The listing builds one solid part. Answer for the finished solid, in the listing's coordinates (mm). A direction names the side the tool comes from. Coordinates: 2 decimals unless noted, no trailing zeros. Order: outer loops, then holes, each group sorted by start corner. A loop starts at its lowest first (then second) coordinate and runs counter-clockwise, first axis right, second up. Notation, with made-up numbers: (48, -38) -> (54, -38) arc R26 ccw to (54, -24) -> close; hole circle Ø10 at (51, -20.75). An arc over 180 degrees is marked (long way). Write item = value, one per line.
from build123d import *

# Parameters (mm, degrees)
F0_W     = 23.8
F0_H     = 14
F0_W_2   = 10.5
F0_H_2   = 12
F1_DEPTH = 5.5
F2_DEPTH = 1.5
F4_DEPTH = 1
F5_R     = 6.5


with BuildPart() as f1:
    # F0 (on Top) → F1 (new body)
    with BuildSketch(Plane.XY):
        with Locations((-0.285932, 2.603267)):
            Rectangle(F0_W, F0_H)
        with Locations((-5.935932, 2.603267)):
            Rectangle(F0_W_2, F0_H_2, mode=Mode.SUBTRACT)
        with BuildLine():
            ThreePointArc((4.464068, 7.655247), (5.464068, 7.753267), (6.464068, 7.655247))
            ThreePointArc((6.464068, 7.655247), (9.443546, 5.87225), (10.614068, 2.603267))
            ThreePointArc((10.614068, 2.603267), (9.443546, -0.665716), (6.464068, -2.448713))
            ThreePointArc((6.464068, -2.448713), (5.464068, -2.546733), (4.464068, -2.448713))
            ThreePointArc((4.464068, -2.448713), (0.314068, 2.603267), (4.464068, 7.655247))
        make_face(mode=Mode.SUBTRACT)
    extrude(amount=F1_DEPTH)

    # F0 (on Top) → F2 (join)
    with BuildSketch(Plane.XY):
        with BuildLine():
            Line((4.464068, 4.655247), (6.464068, 4.655247))
            Line((6.464068, 4.655247), (6.464068, 7.655247))
            ThreePointArc((6.464068, 7.655247), (5.464068, 7.753267), (4.464068, 7.655247))
            Line((4.464068, 7.655247), (4.464068, 4.655247))
        make_face()
        with BuildLine():
            ThreePointArc((4.464068, -2.448713), (5.464068, -2.546733), (6.464068, -2.448713))
            Line((6.464068, -2.448713), (6.464068, 0.551287))
            Line((6.464068, 0.551287), (4.464068, 0.551287))
            Line((4.464068, 0.551287), (4.464068, -2.448713))
        make_face()
    extrude(amount=F2_DEPTH)

    # F3 (on face) → F4 (join)
    with BuildSketch(Plane.XY.offset(5.5)):
        Polygon((-9.185932, 8.603267), (-11.185932, 8.603267), (-11.185932, 6.603267), align=None)
        Polygon((-0.685932, -3.396733), (-0.685932, -1.396733), (-2.685932, -3.396733), align=None)
    extrude(amount=-F4_DEPTH)

    # F5
    f5_edges = [f1.edges().sort_by_distance(p)[0] for p in [
        (11.614068, 9.603267, 2.75),
        (11.614068, -4.396733, 2.75),
    ]]
    fillet(f5_edges, radius=F5_R)


solid = f1.part
Q1. The mould has two halves that part along X. Classify faces 5 (the face through (11.614, 2.6, 2.7)), 6 (the face through (-4, -4.397, 3)), 7 (the face through (-11.186, 3, 3)): released by +X, released by -X, zero draft, split by the parting line, or undercut.
The answers:
face_5 = released by +X
face_6 = zero draft
face_7 = undercut
Q2. Section C-C, the plane z = 4.8 is taken. Give the vertices of the cut face in (x, y), plus the area to 3 significant figures.
The answers:
outline = (-12.19, -4.4) -> (5.11, -4.4) arc R6.5 ccw to (11.61, 2.1) -> (11.61, 3.1) arc R6.5 ccw to (5.11, 9.6) -> (-12.19, 9.6) -> close; hole (-11.19, -3.4) -> (-2.69, -3.4) -> (-0.69, -1.4) -> (-0.69, 8.6) -> (-9.19, 8.6) -> (-11.19, 6.6) -> close; hole (4.46, -2.45) arc R5.15 ccw to (6.46, -2.45) arc R5.15 ccw to (10.61, 2.6) arc R5.15 ccw to (6.46, 7.66) arc R5.15 ccw to (4.46, 7.66) arc R5.15 ccw to start
area = 110 mm2
Q3. A tool of negligible diameter and unlimited length cuts with its end or side. For faces 1 (the face through (9.66, -2.54, 2.79)), 2 (the face through (-0.686, 3, 3)), 3 (the face through (4.464, 6, 1)), 4 (the face through (5, 6, 1.5)), from which of +Z, -Z, +X, -X, +Y, -Y can it reach the whole face along a straight path? Write none if from no direction.
The answers:
face_1 = +Z, -Z, +X, -Y
face_2 = -Z
face_3 = +Z, -Z
face_4 = +Z
Q4. Section B-B, the plane y = 5.25 is taken. Give the vertices of the cut face in (x, z).
The answers:
outline = (-12.19, 0) -> (-11.19, 0) -> (-11.19, 5.5) -> (-12.19, 5.5) -> close; (-0.69, 0) -> (1.05, 0) -> (1.05, 5.5) -> (-0.69, 5.5) -> close; (4.46, 0) -> (6.46, 0) -> (6.46, 1.5) -> (4.46, 1.5) -> close; (9.88, 0) -> (11.25, 0) -> (11.25, 5.5) -> (9.88, 5.5) -> close
Q5. Each of these flat-tipped pins is pushed along its axis until it touches: pin 1 Ø0.8 at (y, z) = (6, 0.5) entering from +X; pin 2 Ø1 at (x, y) = (5, 6) entering from +Z; pin 3 Ø0.6 at (x, y) = (-10, 7.5) entering from -Z. Where does it stop, or does it pass through?
The answers:
pin_1 = 11.12
pin_2 = 1.5
pin_3 = 4.5
Q6. Find the intervals of material crossed by line 1 along X through (y, z) = (2.75, 1.1); line 2 along Y through (x, z) = (-2.75, 4.6); line 3 along X through (y, z) = (-1.75, 4.3), in increasing order.
The answers:
line_1 = -12.19 to -11.19, -0.69 to 0.32, 10.61 to 11.61
line_2 = -4.4 to -3.4, 8.6 to 9.6
line_3 = -12.19 to -11.19, -0.69 to 2.71, 8.22 to 10.35
Q7. Section D-D, the plane y = 8 is taken. Give the vertices of the cut face in (x, z), plus the area to 3 significant figures.
The answers:
outline = (-12.19, 0) -> (-11.19, 0) -> (-11.19, 4.5) -> (-9.79, 4.5) -> (-9.79, 5.5) -> (-12.19, 5.5) -> close; (-0.69, 0) -> (9.39, 0) -> (9.39, 5.5) -> (-0.69, 5.5) -> close
area = 62.3 mm2
Q8. Section A-A, the plane x = -8.25 is taken. Give the vertices of the cut face in (y, z).
The answers:
outline = (-4.4, 0) -> (-3.4, 0) -> (-3.4, 5.5) -> (-4.4, 5.5) -> close; (8.6, 0) -> (9.6, 0) -> (9.6, 5.5) -> (8.6, 5.5) -> close
